from build123d import *

# Parameters (mm, degrees)
SKETCH1_R           = 2.05
BOSS_EXTRUDE1_DEPTH = 14
SKETCH2_R           = 2.05
CUT_EXTRUDE1_DEPTH  = 35.788647574


with BuildPart() as part:
    # Sketch1 → Boss-Extrude1 (new body)
    with BuildSketch(Plane(origin=(0, 0, 0), x_dir=(1, 0, 0), z_dir=(0, 1, 0))):
        with BuildLine():
            Line((-19.55, 0), (-19.55, -3.98647317))
            ThreePointArc((-19.55, -3.98647317), (-18.877985148, -6.048632233), (-17.12, -7.318904715))
            ThreePointArc((-17.12, -7.318904715), (0, -10), (17.12, -7.318904715))
            ThreePointArc((17.12, -7.318904715), (18.877985148, -6.048632233), (19.55, -3.98647317))
            Line((19.55, -3.98647317), (19.55, 0))
            ThreePointArc((19.55, 0), (18.22693576, 3.59659757), (14.888553485, 5.478409687))
            Line((14.888553485, 5.478409687), (8.589900273, 6.5))
            ThreePointArc((8.589900273, 6.5), (7.988389953, 6.839065246), (7.75, 7.487100845))
            Line((7.75, 7.487100845), (7.75, 15.9))
            ThreePointArc((7.75, 15.9), (7.603553391, 16.253553391), (7.25, 16.4))
            Line((7.25, 16.4), (0.75, 16.4))
            Line((0.75, 16.4), (0.75, 4.943429983))
            ThreePointArc((0.75, 4.943429983), (0, -5), (-0.75, 4.943429983))
            Line((-0.75, 4.943429983), (-0.75, 16.4))
            Line((-0.75, 16.4), (-7.25, 16.4))
            ThreePointArc((-7.25, 16.4), (-7.603553391, 16.253553391), (-7.75, 15.9))
            Line((-7.75, 15.9), (-7.75, 7.487100845))
            ThreePointArc((-7.75, 7.487100845), (-7.988389953, 6.839065246), (-8.589900273, 6.5))
            Line((-8.589900273, 6.5), (-14.888553485, 5.478409687))
            ThreePointArc((-14.888553485, 5.478409687), (-18.22693576, 3.59659757), (-19.55, 0))
        make_face()
        with Locations(Location((-14, 0, 0), (0, 0, 270))):
            Circle(SKETCH1_R, mode=Mode.SUBTRACT)
        with Locations(Location((14, 0, 0), (0, 0, 270))):
            Circle(SKETCH1_R, mode=Mode.SUBTRACT)
    extrude(amount=BOSS_EXTRUDE1_DEPTH)

    # Sketch2 → Cut-Extrude1 (cut, through all)
    with BuildSketch(Plane(origin=(7.75, 0, 0), x_dir=(0, 0, -1), z_dir=(1, 0, 0))):
        with Locations((11.9, 7)):
            Circle(SKETCH2_R)
    extrude(amount=-CUT_EXTRUDE1_DEPTH, mode=Mode.SUBTRACT)


solid = part.part
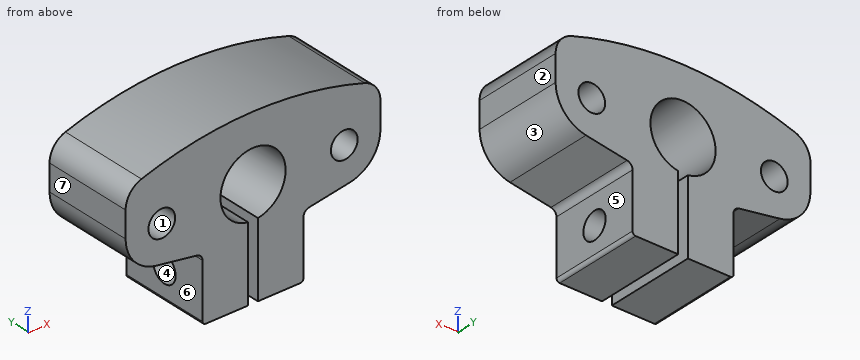
Here's how the part is built. I have some questions about the finished solid (model axes, mm). Face numbers are marked on the shaded views. A direction names the side the tool comes from. Coordinates: 2 decimals unless noted, no trailing zeros. Order: outer loops, then holes, each group sorted by start corner. A loop starts at its lowest first (then second) coordinate and runs counter-clockwise, first axis right, second up. Notation, with made-up numbers: (7.5, -30.75) - (16.5, -30.75) arc R4 ccw to (16.5, -25.75) - close; hole circle Ø1 at (51, 59.25). An arc over 180 degrees is marked (long way). Use CSV: the item, a comma, the result in double quotes. Start each with the question number.
1. Please list where these lines run through material, in increasing order: line 1 (X direction, y = 11.75, z = -10.25); line 2 (Y direction, x = -4.25, z = -11.9); line 3 (X direction, y = 2, z = -0.25). Write a range as from..to.
2. For the marked faces 5, 6 and 7, which set-ups out of +Z, -Z, +X, -X, +Y, -Y let a thin tool reach every point of the face, with its end or its side?
3. Suppose I cut it at A-A on y = 7. Give the number of separate pieces and of enclosed holes in the cut face, then the cut area to 3 significant figures.
4. I'm going to push flat-ended pins straight in: pin 1 (1 mm diameter, centred on y = 10, z = -2.5, fed in from +X); pin 2 (3 mm diameter, centred on y = 2.5, z = -4.5, fed in from +X); pin 3 (5.5 mm diameter, centred on y = 8, z = -11, fed in from -X). Where does each tip first touch, or does it pass through?
5. Suppose I cut it at B-B on x = 4. List the corners of the cut face in (y, z) for me.
6. If we mould it in two halves opening along Z, with no side actions, what happens to the marked faces 1, 2, 3 and 4? For each: +Z half, -Z half, draft (parallel to the pull), parting line (faces both ways), or undercut.
7. Suppose I cut it at C-C on z = -11.9. List the corners of the cut face in (x, y) for me, then the cut area to 3 significant figures.
8. Suppose I cut it at D-D on x = 14. List the corners of the cut face in (y, z) for me.
Output:
1,line 1,"x = -7.75..-0.75, 0.75..7.75"
1,line 2,"y = 0..4.95, 9.05..14"
1,line 3,"x = -19.54..-16.03, -11.97..-4.99, 4.99..11.97, 16.03..19.54"
2,face 5,"-Z, +X, +Y, -Y"
2,face 6,"-Z, -X, +Y, -Y"
2,face 7,"+Z, -Z, -X, +Y, -Y"
3,separate pieces,"3"
3,enclosed holes,"2"
3,area,"543 mm2"
4,pin 1,"stops at x = 19.18"
4,pin 2,"stops at x = 18.67"
4,pin 3,"stops at x = -7.75"
5,outline,"(0, -16.4) - (14, -16.4) - (14, -3) - (0, -3) - close; (0, 3) - (14, 3) - (14, 9.86) - (0, 9.86) - close; hole circle Ø4.1 at (7, -11.9)"
6,face 1,"undercut"
6,face 2,"draft"
6,face 3,"-Z half"
6,face 4,"undercut"
7,outline,"(-7.75, 0) - (-0.75, 0) - (-0.75, 4.95) - (-7.75, 4.95) - close; (-7.75, 9.05) - (-0.75, 9.05) - (-0.75, 14) - (-7.75, 14) - close; (0.75, 0) - (7.75, 0) - (7.75, 4.95) - (0.75, 4.95) - close; (0.75, 9.05) - (7.75, 9.05) - (7.75, 14) - (0.75, 14) - close"
7,area,"139 mm2"
8,outline,"(0, -5.62) - (14, -5.62) - (14, -2.05) - (0, -2.05) - close; (0, 2.05) - (14, 2.05) - (14, 8.22) - (0, 8.22) - close"
